Autodesk Fusion 360 part; units mm, degrees
sketch "スケッチ1" plane through (0, 0, 0) normal (0, 1, 0) x (1, 0, 0)
  arc A0 (77.7618, -166.7606) -> (77.7618, 166.7606) centre (0, 0) ccw
  arc A1 (84.5237, -181.2616) -> (84.5237, 181.2616) centre (0, 0) ccw
  line L0 (84.5237, 181.2616) -> (0, 0)
  line L1 (0, 0) -> (84.5237, -181.2616)
  arc A2 (96, -166.2769) -> (96, 166.2769) centre (0, 0) ccw
  line L2 (96, 166.2769) -> (0, 0)
  line L3 (96, -166.2769) -> (0, 0)
  line L4 (0, 0) -> (192, 0)
  dimension "d1" = 200
  dimension "d2" = 184
  dimension "d3" = 192
  dimension "d4" = 60
  dimension "d5" = 60
  dimension "d6" = 65
  dimension "d8" = 65
extrude "押し出し1" add sketch "スケッチ1" along normal blind 6 contours A0 A1 L0 L1 A2 L2 L3 | A0 A2 L3 L4 | A0 A2 L2 L4
hole "穴1" at (192, 0, 0) at (96, 0, 166.2769) at (96, 0, -166.2769) direction (0, 1, 0) diameter 3.2 end through all
fillet "フィレット1" radius 1 4 edges at (84.5237, 3, 181.2616) (77.7618, 3, 166.7606) (84.5237, 3, -181.2616) (77.7618, 3, -166.7606)
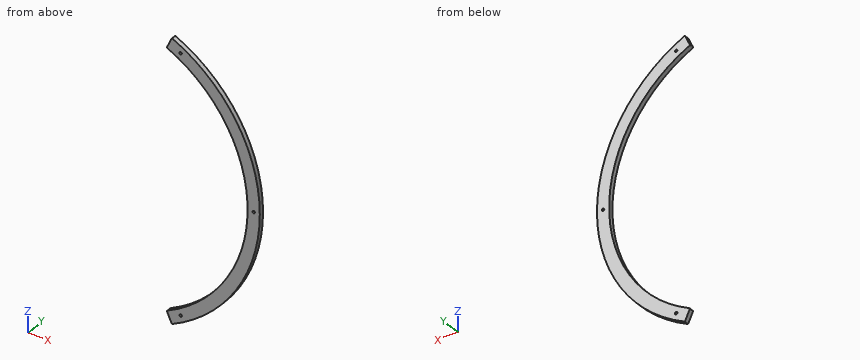
Geometry: final body of the model. Coordinates: model frame, mm. Coordinates: 2 decimals unless noted, no trailing zeros. Order: outer loops, then holes, each group sorted by start corner. A loop starts at its lowest first (then second) coordinate and runs counter-clockwise, first axis right, second up.
1) Section A-A (x = 177.5). Return loops of the section in (y, z).
Result sheet:
outline: (0, -92.16) - (6, -92.16) - (6, -48.47) - (0, -48.47) - close; (0, 48.47) - (6, 48.47) - (6, 92.16) - (0, 92.16) - close
2) Section D-D (z = -76). Return loops of the section in (x, y), then the cut area to 3 significant figures.
Result sheet:
outline: (167.57, 0) - (185, 0) - (185, 6) - (167.57, 6) - close
area: 105 mm2
3) First-contact query: P1, Ø3, axis at y = 4.5, z = 20.5, coming from the +X side; P2, Ø1, axis at x = 102, y = 3, coming from the -Z side. Flat tips, straight axial feed; report the tip coordinate or a pass-through.
Result sheet:
P1: stops at x = 199.1
P2: stops at z = -172.33
4) Section B-B (y = 1.1). Return loops of the section in (x, z).
Result sheet:
outline: (78.18, -167.66) - (84.1, -180.35) arc R1 ccw to (85.43, -180.83) arc R200 ccw to (85.43, 180.83) arc R1 ccw to (84.1, 180.35) - (78.18, 167.66) arc R1 ccw to (78.66, 166.34) arc R184 cw to (78.66, -166.34) arc R1 ccw to start; hole circle Ø3.2 at (96, -166.28); hole circle Ø3.2 at (96, 166.28); hole circle Ø3.2 at (192, 0)
5) Ray query, probe 1 along Z at (x, y) = (96, 3.1); probe 2 along Z at (x, y) = (148, 4.85); probe 3 along Z at (x, y) = (118.5, 4.5). Return the intervals inside material, ascending.
Result sheet:
probe 1: z = -175.45 to -167.88, -164.68 to -156.97, 156.97 to 164.68, 167.88 to 175.45
probe 2: z = -134.52 to -109.33, 109.33 to 134.52
probe 3: z = -161.11 to -140.76, 140.76 to 161.11
6) Section C-C (x = 153). Return loops of the section in (y, z).
Result sheet:
outline: (0, -128.81) - (6, -128.81) - (6, -102.21) - (0, -102.21) - close; (0, 102.21) - (6, 102.21) - (6, 128.81) - (0, 128.81) - close
